Autodesk Inventor part; units mm, degrees
ref_plane "YZ Plane" through (0, 0, 0) normal (1, 0, 0) x (0, 1, 0)
ref_plane "XZ Plane" through (0, 0, 0) normal (0, 1, 0) x (-1, 0, 0)
ref_plane "XY Plane" through (0, 0, 0) normal (0, 0, 1) x (1, 0, 0)
sketch "Schizzo1" plane through (0, 0, 0) normal (0, 1, 0) x (-1, 0, 0)
  circle A0 centre (0, 0) radius 15
  circle A1 centre (0, 0) radius 40
  dimension "d0" = 30
  dimension "d1" = 80
extrude "Estrusione1" add sketch "Schizzo1" against normal blind 34
sketch "Schizzo2" plane through (0, -34, 0) normal (0, -1, 0) x (1, 0, 0)
  circle A0 centre (0, 0) radius 15
  circle A1 centre (0, 0) radius 42.5
  dimension "d4" = 85
extrude "Estrusione2" add sketch "Schizzo2" against normal blind 34
sketch "Schizzo3" plane through (0, -34, 0) normal (0, -1, 0) x (1, 0, 0)
  circle A0 centre (0, 0) radius 34.885
  line L0 (0, 41.5801) -> (0, 0)
  line L1 (0, 0) -> (-42.3383, -3.7041)
  circle A1 centre (0, 0) radius 42.5
  line L2 (42.3383, -3.7041) -> (0, 0)
  point P0 (-34.7523, -3.0404)
  point P1 (34.7523, -3.0404)
  dimension "d7" = 69.77
  dimension "d8" = 95
  dimension "d9" = 95
hole "Foro1" at (-34.7523, -34, -3.0404) at (34.7523, -34, -3.0404) direction (0, 1, 0) diameter 11.4 depth 19.8 tip angle 118
sketch "Schizzo4" plane through (0, -34, 0) normal (0, -1, 0) x (1, 0, 0)
  circle A0 centre (0, 0) radius 34.885
  point P0 (0, 34.885)
  dimension "d17" = 69.77
hole "Foro2" at (0, -34, 34.885) direction (0, 1, 0) diameter 10.262 depth 32 tip angle 118
sketch "Schizzo5" plane through (0, -34, 0) normal (0, -1, 0) x (1, 0, 0)
  circle A0 centre (0, 0) radius 20
  dimension "d25" = 40
extrude "Estrusione3" cut sketch "Schizzo5" against normal blind 34
sketch "Schizzo6" plane through (0, 0, 0) normal (0, 1, 0) x (1, 0, 0)
  circle A0 centre (0, 0) radius 20
  circle A1 centre (0, -34.885) radius 1.8024
  circle A2 centre (0, 0) radius 42.5
extrude "Estrusione4" cut sketch "Schizzo6" against normal blind 2
sketch "Schizzo7" plane through (0, -34, 0) normal (0, -1, 0) x (1, 0, 0)
  circle A0 centre (0, 0) radius 34.885
  circle A1 centre (0, 0) radius 42.5
  dimension "d30" = 69.77
extrude "Estrusione5" cut sketch "Schizzo7" against normal blind 32
properties part number "sfacciatura + tornitura piana interna ed esterna" material "Ferro, Ghisa grigia ASTM A48 Grado 20"
Model file for the job. Use its own axes, mm. Coordinates: 2 decimals unless noted, no trailing zeros. Loops run counter-clockwise (first coordinate to the right, second up) from the corner with the lowest first, then second, coordinate; pieces in that order, holes last. Notation, with made-up numbers: (-23.75, -33) - (7.25, -33) arc R22 ccw to (7.25, 2) - close; hole circle Ø4 at (13, -13). An arc over 180 degrees is marked (long way). Answer as a JSON object with one key per item and string values. Group by question number.
(1) Cut at B-B (z = 15). Give the cut face in (x, y), then the cut area to 3 significant figures.
(2) Flat gauge pins, fed straight in: pin 1 (5 mm diameter, centred on y = -22.5, z = 15.5, fed in from +X); pin 2 (5 mm diameter, centred on y = -26, z = 19, fed in from -X); pin 3 (3 mm diameter, centred on x = -9.5, y = -9.5, fed in from -Z). Where does each tip first touch, or does it go through?
(3) Two-plate mould, pull along X, no slides. Class faces 1 (the face through (33.51, -18.22, -9.7)), 2 (the face through (15, -2, 15)), 3 (the face through (0.108, -17.776, 29.755)): released by +X, released by -X, zero draft, split by the parting line, or undercut.
(4) Cut at D-D (x = -27). Give the cut face in (y, z), then the cut area to 3 significant figures.
(5) Cut at C-C (z = -30). Give the cut face in (x, y).
(6) Cut at A-A (x = 0). Give the cut face in (y, z) (3 decimals), then the cut area to 3 significant figures.
(7) Probe line 1 along Z through (x, y) = (0, -12.5) (3 decimals); line 2 along Z through (x, y) = (-12, -22.5); line 3 along X through (y, z) = (-9, 0) (3 decimals). List the from-to ranges inside material, lowest first.
Geometry says:
{
 "1": {"outline": "(-31.5, -34) - (-13.23, -34) - (-13.23, -2) - (-31.5, -2) - close; (13.23, -34) - (31.5, -34) - (31.5, -2) - (13.23, -2) - close", "area": "1,170 mm^2"},
 "2": {"pin 1": "stops at x = 32.37", "pin 2": "stops at x = -30.74", "pin 3": "stops at z = -33.96"},
 "3": {"face 1": "split by the parting line", "face 2": "zero draft", "face 3": "undercut"},
 "4": {"outline": "(-34, -22.09) - (-2, -22.09) - (-2, 22.09) - (-34, 22.09) - close", "area": "1,410 mm^2"},
 "5": {"outline": "(-17.8, -34) - (17.8, -34) - (17.8, -2) - (-17.8, -2) - close"},
 "6": {"outline": "(-34, -34.885) - (-2, -34.885) - (-2, -20) - (-34, -20) - close; (-34, 20) - (-2, 20) - (-2, 29.754) - (-34, 29.754) - close", "area": "788 mm^2"},
 "7": {"line 1": "z = -34.885 to -20, 20 to 29.754", "line 2": "z = -32.76 to -16, 16 to 32.76", "line 3": "x = -34.885 to -20, 20 to 34.885"}
}
